from build123d import *

# Parameters (mm, degrees)
SKETCH1_R           = 1
BOSS_EXTRUDE1_DEPTH = 2.54
MIRROR2_OUTLINE_R   = 1
MIRROR2_DEPTH       = 2.54


# Read off the part's stored shape, not the designer's step: Mirror2
with BuildPart() as part:
    # Sketch1 → Boss-Extrude1 (new body)
    with BuildSketch(Plane(origin=(0, 0, 0), x_dir=(1, 0, 0), z_dir=(0, 1, 0))):
        with BuildLine():
            Line((0, 22), (0, 15))
            ThreePointArc((0, 15), (-10.606601718, 10.606601718), (-15, 0))
            Line((-15, 0), (-22, 0))
            Line((-22, 0), (-22, 22))
            Line((-22, 22), (0, 22))
        make_face()
        with Locations(Location((-19, 19, 0), (0, 0, 270))):
            Circle(SKETCH1_R, mode=Mode.SUBTRACT)
    extrude(amount=BOSS_EXTRUDE1_DEPTH)

    # Mirror2 outline → Mirror2 (add)
    with BuildSketch(Plane(origin=(0, 0, 0), x_dir=(1, 0, 0), z_dir=(0, 1, 0))):
        with BuildLine():
            Line((22, 22), (0, 22))
            Line((0, 22), (0, 15))
            ThreePointArc((0, 15), (10.606601718, -10.606601718), (-15, 0))
            Line((-15, 0), (-22, 0))
            Line((-22, 0), (-22, -22))
            Line((-22, -22), (22, -22))
            Line((22, -22), (22, 22))
        make_face()
        with Locations((-19, -19)):
            Circle(MIRROR2_OUTLINE_R, mode=Mode.SUBTRACT)
        with Locations((19, -19)):
            Circle(MIRROR2_OUTLINE_R, mode=Mode.SUBTRACT)
        with Locations((19, 19)):
            Circle(MIRROR2_OUTLINE_R, mode=Mode.SUBTRACT)
    extrude(amount=MIRROR2_DEPTH)


solid = part.part
Read the model definition and answer for the solid it produces. Units are mm, in the model's axes. Round coordinates to 2 decimals unless told otherwise and drop trailing zeros. Order: outer loops, then holes, each group sorted by start corner. A loop starts at its lowest first (then second) coordinate and runs counter-clockwise, first axis right, second up. Notation, with made-up numbers: (43.25, -26) - (54.25, -26) arc R25 cw to (54.25, -9) - close; hole circle Ø2 at (38.5, -6). An arc over 180 degrees is marked (long way). Use one line per item in the form item = value. Start each with the question number.
(1) Flat-ended cylindrical pins translate along their axes: pin 1 Ø1.2 at (x, z) = (19, 19) entering from +Y; pin 2 Ø12 at (x, z) = (9, -13.5) entering from -Y. Find the tip coordinate at first contact, or state that the pin passes through.
(2) The part is cut by section D-D (x = 14). Give the vertices of the cut face in (y, z), then the cut area to 3 significant figures.
(3) The part is cut by section A-A (x = 19). Give the vertices of the cut face in (y, z), then the cut area to 3 significant figures.
(4) The part is cut by section B-B (z = 19). Give the vertices of the cut face in (x, y).
(5) Find the intervals of material crossed by line 1 along X through (y, z) = (0.25, -19); line 2 along X through (y, z) = (1.2, 0), in increasing order. Write a range as from..to.
(6) The part is cut by section C-C (y = 1). Give the vertices of the cut face in (x, z).
(7) Determine the mould class of faces 1 (the face through (19, 1, 20)), 2 (the face through (-22, 1, 0)), 3 (the face through (0, 1, 22)) for opening direction X: +X half, -X half, draft (parallel to the pull), parting line (faces both ways), or undercut.
Checked values:
q1.pin_1 = through
q1.pin_2 = 0
q2.outline = (0, -22) - (2.54, -22) - (2.54, -5.39) - (0, -5.39) - close; (0, 5.39) - (2.54, 5.39) - (2.54, 22) - (0, 22) - close
q2.area = 84.4 mm^2
q3.outline = (0, -22) - (2.54, -22) - (2.54, -20) - (0, -20) - close; (0, -18) - (2.54, -18) - (2.54, 18) - (0, 18) - close; (0, 20) - (2.54, 20) - (2.54, 22) - (0, 22) - close
q3.area = 102 mm^2
q4.outline = (-22, 0) - (-20, 0) - (-20, 2.54) - (-22, 2.54) - close; (-18, 0) - (18, 0) - (18, 2.54) - (-18, 2.54) - close; (20, 0) - (22, 0) - (22, 2.54) - (20, 2.54) - close
q5.line_1 = -22..-20, -18..18, 20..22
q5.line_2 = -22..-15, 15..22
q6.outline = (-22, -22) - (22, -22) - (22, 22) - (-22, 22) - close; hole circle Ø2 at (-19, -19); hole circle Ø2 at (-19, 19); hole circle Ø30 at (0, 0); hole circle Ø2 at (19, -19); hole circle Ø2 at (19, 19)
q7.face_1 = undercut
q7.face_2 = -X half
q7.face_3 = draft
